Autodesk Inventor part; units mm, degrees
ref_plane "YZ Plane" through (0, 0, 0) normal (1, 0, 0) x (0, 1, 0)
ref_plane "XZ Plane" through (0, 0, 0) normal (0, 1, 0) x (-1, 0, 0)
ref_plane "XY Plane" through (0, 0, 0) normal (0, 0, 1) x (1, 0, 0)
sketch "スケッチ1" plane through (0, 0, 0) normal (0, 0, 1) x (1, 0, 0)
  circle A0 centre (0, 0) radius 10.5 construction
  line L0 (-13.5, 28) -> (13.5, 28) construction
  line L1 (13.5, 28) -> (13.5, 1) construction
  line L2 (13.5, 1) -> (-13.5, 1) construction
  line L3 (-13.5, 1) -> (-13.5, 28) construction
  line L4 (-13.5, 28) -> (13.5, 1) construction
  line L5 (13.5, 28) -> (-13.5, 1) construction
  line L6 (-13.5, 14.5) -> (13.5, 14.5) construction
  line L7 (0, 28) -> (0, 1) construction
  circle A1 centre (-13.5, 28) radius 1.35
  circle A2 centre (-13.5, 1) radius 2.4 construction
  circle A3 centre (-13.5, 28) radius 2.4 construction
  line L8 (-19.75, 30.4) -> (19.75, 30.4)
  line L9 (-21.75, 25.4) -> (-21.75, 3.6)
  line L10 (-21.75, 25.4) -> (-19.75, 25.4)
  arc A4 (-19.75, 25.4) -> (-19.75, 27.5) centre (-19.75, 26.45) ccw
  line L11 (-19.75, 27.5) -> (-19.75, 30.4)
  line L12 (-21.75, 3.6) -> (-19.75, 3.6)
  arc A5 (-19.75, 1.5) -> (-19.75, 3.6) centre (-19.75, 2.55) ccw
  line L13 (-19.75, 1.5) -> (-19.75, -1.4)
  line L14 (-19.75, -1.4) -> (-10.6584, -1.4)
  line L15 (21.75, 25.4) -> (21.75, 3.6)
  arc A6 (19.75, 27.5) -> (19.75, 25.4) centre (19.75, 26.45) ccw
  line L16 (19.75, 27.5) -> (19.75, 30.4)
  arc A7 (19.75, 3.6) -> (19.75, 1.5) centre (19.75, 2.55) ccw
  line L17 (21.75, 3.6) -> (19.75, 3.6)
  line L18 (19.75, 1.5) -> (19.75, -1.4)
  line L19 (19.75, -1.4) -> (10.6584, -1.4)
  line L20 (21.75, 25.4) -> (19.75, 25.4)
  arc A8 (10.6584, -1.4) -> (-10.6584, -1.4) centre (0, 0) ccw
  circle A9 centre (13.5, 28) radius 1.35
  line L21 (10.5606, 27.4) -> (-10.5606, 27.4)
  arc A10 (-13.5, 25) -> (-10.5606, 27.4) centre (-13.5, 28) ccw
  line L22 (-13.5, 25) -> (-16.75, 25)
  line L23 (-16.75, 25) -> (-16.75, 4)
  arc A11 (12.1063, 4) -> (-12.1063, 4) centre (0, 0) ccw
  line L24 (-16.75, 4) -> (-12.1063, 4)
  arc A12 (10.5606, 27.4) -> (13.5, 25) centre (13.5, 28) ccw
  line L25 (13.5, 25) -> (16.75, 25)
  line L26 (16.75, 25) -> (16.75, 4)
  line L27 (16.75, 4) -> (12.1063, 4)
  line L28 (-13.5, 2.35) -> (-13.5, 2.35)
  line L29 (-13.5, -0.35) -> (-13.5, -0.35)
  arc A13 (-13.5, -0.35) -> (-13.5, 2.35) centre (-13.5, 1) ccw
  arc A14 (-13.5, 2.35) -> (-13.5, -0.35) centre (-13.5, 1) ccw
  line L30 (13.5, -0.35) -> (13.5, -0.35)
  arc A15 (13.5, 2.35) -> (13.5, -0.35) centre (13.5, 1) ccw
  arc A16 (13.5, -0.35) -> (13.5, 2.35) centre (13.5, 1) ccw
  line L31 (13.5, 2.35) -> (13.5, 2.35)
  point P0 (0, 14.5)
  dimension "d0" = 21
  dimension "d3" = 27
  dimension "d4" = 27
  dimension "d6" = 1
  dimension "d7" = 4.8
  dimension "d8" = 2
  dimension "d9" = 1.05
  dimension "d10" = 39.5
  dimension "d11" = 5
  dimension "d12" = 5
  dimension "d13" = 21.8
  dimension "d14" = 0.25
  dimension "d15" = 3
  dimension "d16" = 3
  dimension "d17" = 3
  dimension "d18" = 2
  dimension "d24" = 2.7
  dimension "d25" = 1.35
  dimension "d26" = 0
extrude "押し出し1" add sketch "スケッチ1" along normal blind 2
fillet "フィレット1" radius 2 2 edges at (-10.6584, -1.4, 1) (10.6584, -1.4, 1)
fillet "フィレット2" radius 2 8 edges at (-16.75, 4, 1) (-16.75, 25, 1) (-10.5606, 27.4, 1) (10.5606, 27.4, 1) (16.75, 25, 1) (16.75, 4, 1) (12.1063, 4, 1) (-12.1063, 4, 1)
equation "\"d25\" = 0.5 * d24"
properties part number "Ankle_back_frame" material "アルミニウム 2014-T4"
Work out the finished part from the listing and answer in its coordinate system (mm). A direction names the side the tool comes from. Round coordinates to 2 decimals unless told otherwise and drop trailing zeros. Write each loop counter-clockwise with the first axis right and the second up, starting at its lowest first coordinate (ties: lowest second). Pieces come first, ordered by that corner, then holes. Notation, with made-up numbers: (74.5, -39.75) -> (89.5, -39.75) arc R34 cw to (89.5, -1.75) -> close; hole circle Ø1 at (11, 81). An arc over 180 degrees is marked (long way). Write each question's results on one line, items separated by ' | '.
1) Flat-ended cylindrical pins translate along their axes: pin 1 (1 mm diameter, centred on y = -0.5, z = 1, fed in from -X); pin 2 (8 mm diameter, centred on x = -1.5, y = 12.5, fed in from -Z); pin 3 (0.6 mm diameter, centred on y = 29.5, z = 1, fed in from +X); pin 4 (0.6 mm diameter, centred on x = 21, z = 1, fed in from +Y). Find the tip coordinate at first contact, or state that the pin passes through.
Findings:
pin 1: stops at x = -19.75 | pin 2: stops at z = 0 | pin 3: stops at x = 19.75 | pin 4: stops at y = 25.4
2) The part is cut by section A-A (y = 16.5). Write down the section's boundary in (x, z), and give its area (3 significant figures).
Findings:
outline: (-21.75, 0) -> (-16.75, 0) -> (-16.75, 2) -> (-21.75, 2) -> close; (16.75, 0) -> (21.75, 0) -> (21.75, 2) -> (16.75, 2) -> close | area: 20.0 mm²
3) The part is cut by section D-D (z = 1.7). State how many separate pieces and enclosed holes the cut face has, and give its area (3 significant figures).
Findings:
separate pieces: 1 | enclosed holes: 5 | area: 502 mm²
4) Which of the six approach directions +Z, -Z, +X, -X, +Y, -Y give full straight-line access (tool end or side, diameter ignored) to faces 1 (the flat face through (21, 3.6, 1)), 2 (the cylindrical face through (18.7, 26.4, 1)), 3 (the cylindrical face through (-16.15, 24.43, 1.01)), 4 (the cylindrical face through (11.34, -0.83, 1.01))?
Findings:
face 1: +Z, -Z, +X, -Y | face 2: +Z, -Z, +X | face 3: +Z, -Z | face 4: +Z, -Z, -Y
5) For a pull along Y with two mould halves and no side action, classify faces 5 (the cylindrical face through (-11.37, -0.86, 1.01)), 6 (the cylindrical face through (18.7, 2.5, 1)), 7 (the flat face through (-21, 25.4, 1)), 8 (the flat face through (19.75, 29, 1)) as +Y half, -Y half, draft (parallel to the pull), parting line (faces both ways), or undercut.
Findings:
face 5: -Y half | face 6: undercut | face 7: +Y half | face 8: draft
6) The part is cut by section B-B (y = 28). Write down the section's boundary in (x, z), and give its area (3 significant figures).
Findings:
outline: (-19.75, 0) -> (-14.85, 0) -> (-14.85, 2) -> (-19.75, 2) -> close; (-12.15, 0) -> (12.15, 0) -> (12.15, 2) -> (-12.15, 2) -> close; (14.85, 0) -> (19.75, 0) -> (19.75, 2) -> (14.85, 2) -> close | area: 68.2 mm²
7) The part is cut by section C-C (x = 4.5). Write down the section's boundary in (y, z), and give its area (3 significant figures).
Findings:
outline: (9.76, 0) -> (11.93, 0) -> (11.93, 2) -> (9.76, 2) -> close; (27.4, 0) -> (30.4, 0) -> (30.4, 2) -> (27.4, 2) -> close | area: 10.3 mm²
8) Consider line 1 along Y through (x, z) = (13.5, 1.5); line 2 along X through (y, z) = (16.5, 0.55); line 3 along Y through (x, z) = (-14.5, 1.05). Determine where each line is inside the solid, lowest interval first. Write a range as [from, to].
Findings:
line 1: y = [-1.4, -0.35], [2.35, 4], [25, 26.65], [29.35, 30.4] | line 2: x = [-21.75, -16.75], [16.75, 21.75] | line 3: y = [-1.4, 0.09], [1.91, 4], [25, 27.09], [28.91, 30.4]
